from build123d import *

# Parameters (mm, degrees)
SKETCH2_W           = 4
SKETCH2_H           = 4
SKETCH2_W_2         = 84
SKETCH2_H_2         = 56.5
BOSS_EXTRUDE1_DEPTH = 4
SKETCH2_3_W         = 4
SKETCH2_3_H         = 4
BOSS_EXTRUDE2_DEPTH = 21
CUT_EXTRUDE1_DEPTH  = 10


with BuildPart() as part:
    # Sketch2 → Boss-Extrude1 (new body)
    with BuildSketch(Plane(origin=(0, 0, 0), x_dir=(1, 0, 0), z_dir=(0, 1, 0))):
        Polygon((-42.970842333, 37.287257019), (-42.970842333, 33.287257019), (-38.970842333, 33.287257019), (49.029157667, 33.287257019), (49.029157667, -27.212742981), (49.029157667, -31.212742981), (53.029157667, -31.212742981), (53.029157667, 37.287257019), align=None)
        with Locations((51.029157667, -33.212742981)):
            Rectangle(SKETCH2_W, SKETCH2_H)
        Polygon((-42.970842333, -31.212742981), (-42.970842333, 29.287257019), (-42.970842333, 33.287257019), (-46.970842333, 33.287257019), (-46.970842333, -35.212742981), (49.029157667, -35.212742981), (49.029157667, -31.212742981), (45.029157667, -31.212742981), align=None)
        with Locations((3.029157667, 1.037257019)):
            Rectangle(SKETCH2_W_2, SKETCH2_H_2)
        with Locations((-44.970842333, 35.287257019)):
            Rectangle(SKETCH2_W, SKETCH2_H)
        with Locations((-40.970842333, 31.287257019)):
            Rectangle(SKETCH2_W, SKETCH2_H)
        Polygon((-38.970842333, 33.287257019), (-38.970842333, 29.287257019), (45.029157667, 29.287257019), (45.029157667, -27.212742981), (49.029157667, -27.212742981), (49.029157667, 33.287257019), align=None)
        Polygon((-38.970842333, 29.287257019), (-42.970842333, 29.287257019), (-42.970842333, -31.212742981), (45.029157667, -31.212742981), (45.029157667, -27.212742981), (-38.970842333, -27.212742981), align=None)
        with Locations((47.029157667, -29.212742981)):
            Rectangle(SKETCH2_W, SKETCH2_H)
    extrude(amount=BOSS_EXTRUDE1_DEPTH)

    # Sketch2_3 → Boss-Extrude2 (add)
    with BuildSketch(Plane(origin=(0, 0, 0), x_dir=(1, 0, 0), z_dir=(0, 1, 0))):
        Polygon((-38.970842333, 33.287257019), (-38.970842333, 29.287257019), (45.029157667, 29.287257019), (45.029157667, -27.212742981), (49.029157667, -27.212742981), (49.029157667, 33.287257019), align=None)
        with Locations((-40.970842333, 31.287257019)):
            Rectangle(SKETCH2_3_W, SKETCH2_3_H)
        Polygon((-38.970842333, 29.287257019), (-42.970842333, 29.287257019), (-42.970842333, -31.212742981), (45.029157667, -31.212742981), (45.029157667, -27.212742981), (-38.970842333, -27.212742981), align=None)
        with Locations((47.029157667, -29.212742981)):
            Rectangle(SKETCH2_3_W, SKETCH2_3_H)
    extrude(amount=BOSS_EXTRUDE2_DEPTH)

    # Sketch3 → Cut-Extrude1 (cut)
    with BuildSketch(Plane.XY.offset(31.212742981)):
        Polygon((3.029157667, 21), (3.029157667, 12.5), (8.529157667, 11.483695652), (8.529157667, 21), align=None)
        Polygon((-2.470842333, 21), (-2.470842333, 13.516304348), (3.029157667, 12.5), (3.029157667, 21), align=None)
        Polygon((3.029157667, 12.5), (-2.470842333, 13.516304348), (-2.470842333, 4), (8.529157667, 4), (8.529157667, 11.483695652), align=None)
    extrude(amount=-CUT_EXTRUDE1_DEPTH, mode=Mode.SUBTRACT)


solid = part.part
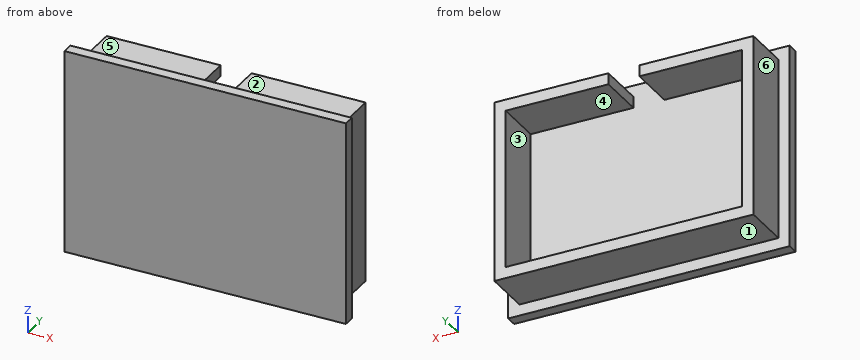
Can you work these out from the model? Positions are in its coordinate system, mm. Face numbers are marked on the shaded views. A direction names the side the tool comes from. Give positions to 0.01 mm unless a question says otherwise; leave off trailing zeros. Order: outer loops, then holes, each group sorted by start corner. A loop starts at its lowest first (then second) coordinate and runs counter-clockwise, first axis right, second up. Notation, with made-up numbers: M 64.25,82.5 L 72.25,82.5 A29 ccw 72.25,103.5 Z; hole C -38,63.25 d7. An arc over 180 degrees is marked long. One line per question, with ' | ' between items.
Item 1: Suppose I cut it at A-A, the plane x = 41. Write out the boundary of the cut face in (y, z).
Answer block:
outline: M 0,-37.29 L 4,-37.29 L 4,-33.29 L 21,-33.29 L 21,-29.29 L 4,-29.29 L 4,27.21 L 21,27.21 L 21,31.21 L 4,31.21 L 4,35.21 L 0,35.21 Z
Item 2: Suppose I cut it at B-B, the plane y = 6.25. Write out the boundary of the cut face in (x, z).
Answer block:
outline: M -42.97,-33.29 L 49.03,-33.29 L 49.03,31.21 L 8.53,31.21 L 8.53,27.21 L 45.03,27.21 L 45.03,-29.29 L -38.97,-29.29 L -38.97,27.21 L -2.47,27.21 L -2.47,31.21 L -42.97,31.21 Z
Item 3: Please list where these lines run through material, in increasing order: L1, parallel to Z at x = 39.5, y = 9.5; L2, parallel to X at y = 15.5, z = 20; L3, parallel to Y at x = 24, z = 19.
Answer block:
L1: z = -33.29 to -29.29, 27.21 to 31.21 | L2: x = -42.97 to -38.97, 45.03 to 49.03 | L3: y = 0 to 4
Item 4: Suppose I cut it at C-C, the plane x = 1.5. Write out the boundary of the cut face in (y, z), then the cut area to 3 significant figures.
Answer block:
outline: M 0,-37.29 L 4,-37.29 L 4,-33.29 L 21,-33.29 L 21,-29.29 L 4,-29.29 L 4,35.21 L 0,35.21 Z | area: 358 mm2
Item 5: I'm going to push flat-ended pins straight in: pin 1 Ø5 at (y, z) = (14, 14.5) entering from -X; pin 2 Ø8.5 at (x, y) = (-2, 12.5) entering from -Z; pin 3 Ø8.5 at (x, y) = (16, 15) entering from +Z. Where does each tip first touch, or does it pass through?
Answer block:
pin 1: stops at x = -42.97 | pin 2: stops at z = -33.29 | pin 3: stops at z = 31.21
Item 6: We'd pull the mould along Z, two halves only. Please class the marked faces 4, 5 and 6: released by +Z, released by -Z, zero draft, split by the parting line, or undercut.
Answer block:
face 4: undercut | face 5: released by +Z | face 6: zero draft
Item 7: For the marked faces 1, 2 and 3, which set-ups out of +Z, -Z, +X, -X, +Y, -Y let a thin tool reach every point of the face, with its end or its side?
Answer block:
face 1: -Z, +X, -X, +Y | face 2: +Z, +X, -X, +Y | face 3: +Y
